The listing builds one solid part. Answer for the finished solid, in the listing's coordinates (mm). Face numbers are marked on the shaded views. Coordinates: 2 decimals unless noted, no trailing zeros. Loops run counter-clockwise (first coordinate to the right, second up) from the corner with the lowest first, then second, coordinate; pieces in that order, holes last. Notation, with made-up numbers: M 89,22 L 137,22 A12 ccw 137,44 Z; hole C -3,-16.5 d5. An arc over 180 degrees is marked long. Answer as a JSON object with one key per item and string values. Group by question number.
1. Determine the mould class of the marked faces 1, 2, 3 and 4 for opening direction Y: released by +Y, released by -Y, zero draft, split by the parting line, or undercut.
2. Straight lines are drawn through the part: L1, parallel to Z at x = 0, y = -13.5; L2, parallel to X at y = -14.2, z = 7.75; L3, parallel to X at y = -9, z = 10.25. For each, find the intervals that lie inside material, in ascending order.
3. A cutting plane is placed at A-A on y = 0. Give the vertices of the cut face in (x, z).
4. A cutting plane is placed at C-C on z = 3. Give the vertices of the cut face in (x, y), and give its area (3 significant figures).
5. A cutting plane is placed at B-B on x = -7. Give the vertices of the cut face in (y, z), and give its area (3 significant figures).
6. A cutting plane is placed at D-D on y = 13. Give the vertices of the cut face in (x, z).
7. Given pin 1 (1.5 mm diameter, centred on y = 6, z = 7, fed in from +X); pin 2 (5 mm diameter, centred on y = 13.5, z = 3.5, fed in from -X); pin 3 (2 mm diameter, centred on y = -10.5, z = 5, fed in from +X), each flat-ended and moving along its own axis, determine where each tip first touches the part or whether it passes through.
from build123d import *

# Parameters (mm, degrees)
SKETCH1_R                    = 10
BOSS_EXTRUDE1_DEPTH          = 15.5
F_2_0_2_DIAMETER_HOLE1_D     = 2
F_2_0_2_DIAMETER_HOLE1_DEPTH = 2
F_2_0_2_DIAMETER_HOLE1_TIP   = 0.600860619


with BuildPart() as part:
    # Sketch1 → Boss-Extrude1 (new body)
    with BuildSketch(Plane.XY):
        with BuildLine():
            Line((-10.84, -14.991477579), (10.84, -14.991477579))
            ThreePointArc((10.84, -14.991477579), (0, 18.5), (-10.84, -14.991477579))
        make_face()
        Circle(SKETCH1_R, mode=Mode.SUBTRACT)
    extrude(amount=BOSS_EXTRUDE1_DEPTH)

    # Ø2.0 (2) Diameter Hole1
    with Locations(Plane(origin=(0, -14.991477579, 0), x_dir=(-1, 0, 0), z_dir=(0, -1, 0))):
        with Locations((0, -7.75)):
            Hole(F_2_0_2_DIAMETER_HOLE1_D / 2, depth=F_2_0_2_DIAMETER_HOLE1_DEPTH)
            with Locations((0, 0, -(F_2_0_2_DIAMETER_HOLE1_DEPTH + F_2_0_2_DIAMETER_HOLE1_TIP / 2))):  # 118° drill point
                Cone(0, F_2_0_2_DIAMETER_HOLE1_D / 2, F_2_0_2_DIAMETER_HOLE1_TIP, mode=Mode.SUBTRACT)


solid = part.part
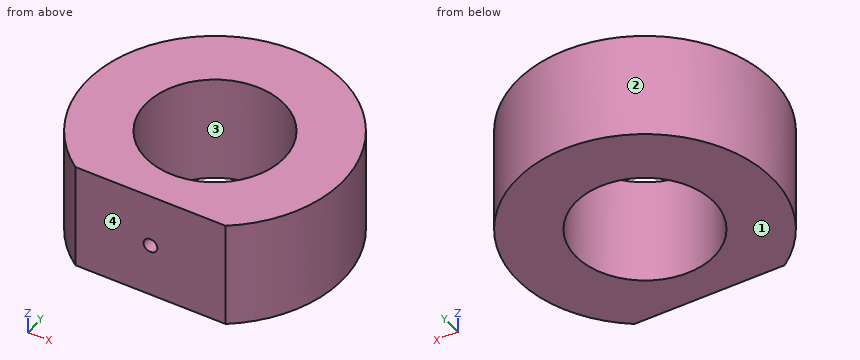
From the geometry:
{
 "1": {"face 1": "zero draft", "face 2": "split by the parting line", "face 3": "undercut", "face 4": "released by -Y"},
 "2": {"L1": "z = 0 to 6.75, 8.75 to 15.5", "L2": "x = -11.86 to -1, 1 to 11.86", "L3": "x = -16.16 to -4.36, 4.36 to 16.16"},
 "3": {"outline": "M -18.5,0 L -10,0 L -10,15.5 L -18.5,15.5 Z; M 10,0 L 18.5,0 L 18.5,15.5 L 10,15.5 Z"},
 "4": {"outline": "M -10.84,-14.99 L 10.84,-14.99 A18.5 ccw long Z; hole C 0,0 d20", "area": "709 mm²"},
 "5": {"outline": "M -14.99,0 L -7.14,0 L -7.14,15.5 L -14.99,15.5 Z; M 7.14,0 L 17.12,0 L 17.12,15.5 L 7.14,15.5 Z", "area": "276 mm²"},
 "6": {"outline": "M -13.16,0 L 13.16,0 L 13.16,15.5 L -13.16,15.5 Z"},
 "7": {"pin 1": "stops at x = 17.74", "pin 2": "stops at x = -14.87", "pin 3": "stops at x = 15.87"}
}
